Source: CAD feature listing. Evaluate the final solid. Frame: model axes, mm. A direction names the side the tool comes from. Coordinates: 2 decimals unless noted, no trailing zeros. Write each loop counter-clockwise with the first axis right and the second up, starting at its lowest first coordinate (ties: lowest second). Pieces come first, ordered by that corner, then holes. Notation, with made-up numbers: (25, -21) - (80, -21) arc R20 cw to (80, -3) - close; hole circle Ø2 at (42, 11). An arc over 180 degrees is marked (long way). One line per question, with ' | ' between items. Start each with the question number.
Q1. Cut plane D-D, the plane y = 1.1. Give the number of separate pieces and of enclosed holes in the cut face, plus the area to 3 significant figures.
Q2. Cut plane A-A, the plane z = 39. Return loops of the section in (x, y).
Q3. Line query: line 1 (X direction, y = 0.65, z = -74); line 2 (Z direction, x = 98, y = 1.5); line 3 (Z direction, x = -50.5, y = 2.4). Output: solid intervals per line, ascending.
Q4. Cut plane B-B, the plane z = -45. Return loops of the section in (x, y).
Q5. Access query for faces 1 (the face through (-26.74, 1.52, -95.9)), 2 (the face through (35.933, 1.521, -43.116)), 3 (the face through (22, 0, -5)). Directions: +Z, -Z, +X, -X, +Y, -Y. A direction counts if a zero-diameter tool reaches every point of the face in a straight line with its end or side. Return the directions, or none.
Q6. Cut plane C-C, the plane x = -64. Return loops of the section in (y, z), plus the area to 3 significant figures.
Q7. Draft query along Z for faces 4 (the face through (115.972, 1.521, 65.502)), 5 (the face through (68.61, 1.52, 89.45)), 6 (the face through (22, 3, -5)). Return one class per face: +Z half, -Z half, draft (parallel to the pull), parting line (faces both ways), or undercut.
Q8. Contact query for flat-ended pins moving along their axis: P1, Ø1.5, axis at x = 21, y = 1.5, coming from the -Z side; P2, Ø8.5, axis at x = -48.36, z = 94.35, coming from the -Y side; P3, Ø0.9, axis at x = 20.5, y = 1.5, coming from the +Z side. Output: stop coordinate, or through.
```python
from build123d import *

# Parameters (mm, degrees)
BOSS_EXTRUDE1_DEPTH = 3
BOSS_EXTRUDE2_DEPTH = 2
CUT_EXTRUDE4_DEPTH  = 167.076115532
SKETCH3_R           = 2.6
CUT_EXTRUDE5_DEPTH  = 167.076115532
CUT_EXTRUDE7_DEPTH  = 167.076115532
SKETCH11_R          = 1.6
CUT_EXTRUDE10_DEPTH = 10
SKETCH12_R          = 2.6
CUT_EXTRUDE12_DEPTH = 10
CUT_EXTRUDE13_DEPTH = 167.076115532


with BuildPart() as part:
    # Sketch1 → Boss-Extrude1 (new body)
    with BuildSketch(Plane(origin=(0, 0, 0), x_dir=(1, 0, 0), z_dir=(0, 1, 0))):
        Polygon((-59.316686906, 108.225499677), (101.185838411, 108.225499677), (125.934575753, 83.476762335), (125.934575753, -77.025762982), (101.185838411, -101.774500323), (-59.316686906, -101.774500323), (-84.065424247, -77.025762982), (-84.065424247, 83.476762335), align=None)
    extrude(amount=BOSS_EXTRUDE1_DEPTH)

    # Sketch2 → Boss-Extrude2 (add)
    with BuildSketch(Plane(origin=(0, 3, 0), x_dir=(1, 0, 0), z_dir=(0, 1, 0))):
        Polygon((-84.065424247, -77.025762982), (-45.174551282, -38.134890016), (-20.425813941, -62.883627358), (-59.316686906, -101.774500323), align=None)
        Polygon((125.934575753, -77.025762982), (93.880849872, -37.104770943), (66.751068905, -58.888061335), (101.185838411, -101.774500323), align=None)
        Polygon((101.185838411, 108.225499677), (62.16108336, 69.955487183), (86.665825958, 44.96747398), (125.934575753, 83.476762335), align=None)
        Polygon((-59.316686906, 108.225499677), (-24.100270952, 65.978558399), (-50.874640527, 43.659845911), (-84.065424247, 83.476762335), align=None)
    extrude(amount=-BOSS_EXTRUDE2_DEPTH)

    # Sketch7 → Cut-Extrude4 (cut, through all)
    with BuildSketch(Plane(origin=(0, 3, 0), x_dir=(1, 0, 0), z_dir=(0, 1, 0))):
        with BuildLine():
            ThreePointArc((-1.565424247, -17.674500323), (-2.696795097, -20.405871173), (0.034575753, -19.274500323))
            Line((0.034575753, -19.274500323), (-1.565424247, -19.274500323))
            Line((-1.565424247, -19.274500323), (-1.565424247, -17.674500323))
        make_face()
        with BuildLine():
            Line((-1.565424247, -19.274500323), (0.034575753, -19.274500323))
            ThreePointArc((0.034575753, -19.274500323), (-0.434053398, -18.143129473), (-1.565424247, -17.674500323))
            Line((-1.565424247, -17.674500323), (-1.565424247, -19.274500323))
        make_face()
        with BuildLine():
            ThreePointArc((43.434575753, -17.674500323), (42.303204903, -18.143129473), (41.834575753, -19.274500323))
            Line((41.834575753, -19.274500323), (43.434575753, -19.274500323))
            Line((43.434575753, -19.274500323), (43.434575753, -17.674500323))
        make_face()
        with BuildLine():
            Line((43.434575753, -19.274500323), (41.834575753, -19.274500323))
            ThreePointArc((41.834575753, -19.274500323), (43.434575753, -20.874500323), (45.034575753, -19.274500323))
            ThreePointArc((45.034575753, -19.274500323), (44.565946602, -18.143129473), (43.434575753, -17.674500323))
            Line((43.434575753, -17.674500323), (43.434575753, -19.274500323))
        make_face()
        with BuildLine():
            ThreePointArc((45.034575753, 25.725499677), (43.434575753, 27.325499677), (41.834575753, 25.725499677))
            Line((41.834575753, 25.725499677), (43.434575753, 25.725499677))
            Line((43.434575753, 25.725499677), (43.434575753, 24.125499677))
            ThreePointArc((43.434575753, 24.125499677), (44.565946602, 24.594128827), (45.034575753, 25.725499677))
        make_face()
        with BuildLine():
            Line((43.434575753, 25.725499677), (41.834575753, 25.725499677))
            ThreePointArc((41.834575753, 25.725499677), (42.303204903, 24.594128827), (43.434575753, 24.125499677))
            Line((43.434575753, 24.125499677), (43.434575753, 25.725499677))
        make_face()
        with BuildLine():
            ThreePointArc((-1.565424247, 24.125499677), (-0.434053398, 24.594128827), (0.034575753, 25.725499677))
            Line((0.034575753, 25.725499677), (-1.565424247, 25.725499677))
            Line((-1.565424247, 25.725499677), (-1.565424247, 24.125499677))
        make_face()
        with BuildLine():
            Line((-1.565424247, 25.725499677), (0.034575753, 25.725499677))
            ThreePointArc((0.034575753, 25.725499677), (-2.696795097, 26.856870527), (-1.565424247, 24.125499677))
            Line((-1.565424247, 24.125499677), (-1.565424247, 25.725499677))
        make_face()
    extrude(amount=-CUT_EXTRUDE4_DEPTH, mode=Mode.SUBTRACT)

    # Sketch3 → Cut-Extrude5 (cut, through all)
    with BuildSketch(Plane(origin=(0, 3, 0), x_dir=(1, 0, 0), z_dir=(0, 1, 0))):
        with Locations(Location((-27.143328362, 79.587675039, 0), (0, 0, 270))):
            Circle(SKETCH3_R)
        with Locations(Location((-55.427599609, 51.303403791, 0), (0, 0, 270))):
            Circle(SKETCH3_R)
        with Locations(Location((-76.640803045, 72.516607227, 0), (0, 0, 270))):
            Circle(SKETCH3_R)
        with Locations(Location((-48.356531798, 100.800878474, 0), (0, 0, 270))):
            Circle(SKETCH3_R)
        with Locations(Location((118.50995455, 72.516607227, 0), (0, 0, 90))):
            Circle(SKETCH3_R)
        with Locations(Location((97.296751114, 51.303403791, 0), (0, 0, 90))):
            Circle(SKETCH3_R)
        with Locations(Location((69.012479867, 79.587675039, 0), (0, 0, 90))):
            Circle(SKETCH3_R)
        with Locations(Location((90.225683303, 100.800878474, 0), (0, 0, 90))):
            Circle(SKETCH3_R)
        with Locations(Location((97.296751114, -44.852404438, 0), (0, 0, 270))):
            Circle(SKETCH3_R)
        with Locations(Location((118.50995455, -66.065607873, 0), (0, 0, 270))):
            Circle(SKETCH3_R)
        with Locations(Location((90.225683303, -94.349879121, 0), (0, 0, 270))):
            Circle(SKETCH3_R)
        with Locations(Location((69.012479867, -73.136675685, 0), (0, 0, 270))):
            Circle(SKETCH3_R)
        with Locations(Location((-27.143328362, -73.136675685, 0), (0, 0, 90))):
            Circle(SKETCH3_R)
        with Locations(Location((-55.427599609, -44.852404438, 0), (0, 0, 90))):
            Circle(SKETCH3_R)
        with Locations(Location((-76.640803045, -66.065607873, 0), (0, 0, 90))):
            Circle(SKETCH3_R)
        with Locations(Location((-48.356531798, -94.349879121, 0), (0, 0, 90))):
            Circle(SKETCH3_R)
    extrude(amount=-CUT_EXTRUDE5_DEPTH, mode=Mode.SUBTRACT)

    # Sketch9 → Cut-Extrude7 (cut, through all)
    with BuildSketch(Plane(origin=(0, 3, 0), x_dir=(1, 0, 0), z_dir=(0, 1, 0))):
        Polygon((-14.065424247, 83.225499677), (55.934575753, 83.225499677), (80.934575753, 108.225499677), (-39.065424247, 108.225499677), align=None)
        Polygon((-14.065424247, -76.774500323), (-39.065424247, -101.774500323), (80.934575753, -101.774500323), (55.934575753, -76.774500323), align=None)
    extrude(amount=-CUT_EXTRUDE7_DEPTH, mode=Mode.SUBTRACT)

    # Sketch11 → Cut-Extrude10 (cut)
    with BuildSketch(Plane(origin=(0, 3, 0), x_dir=(1, 0, 0), z_dir=(0, 1, 0))):
        with Locations(Location((-77.065424247, 17.565499677, 0), (0, 0, 270))):
            Circle(SKETCH11_R)
        with Locations(Location((-77.065424247, -11.114500323, 0), (0, 0, 270))):
            Circle(SKETCH11_R)
        with Locations(Location((-48.385424247, 17.565499677, 0), (0, 0, 270))):
            Circle(SKETCH11_R)
        with Locations(Location((-48.385424247, -11.114500323, 0), (0, 0, 90))):
            Circle(SKETCH11_R)
    extrude(amount=-CUT_EXTRUDE10_DEPTH, mode=Mode.SUBTRACT)

    # Sketch12 → Cut-Extrude12 (cut)
    with BuildSketch(Plane(origin=(0, 3, 0), x_dir=(1, 0, 0), z_dir=(0, 1, 0))):
        with Locations(Location((-34.065424247, 3.225499677, 0), (0, 0, 270))):
            Circle(SKETCH12_R)
        with Locations(Location((20.934575753, -51.774500323, 0), (0, 0, 270))):
            Circle(SKETCH12_R)
        with Locations(Location((75.934575753, 3.225499677, 0), (0, 0, 270))):
            Circle(SKETCH12_R)
        with Locations(Location((20.934575753, 58.225499677, 0), (0, 0, 270))):
            Circle(SKETCH12_R)
    extrude(amount=-CUT_EXTRUDE12_DEPTH, mode=Mode.SUBTRACT)

    # Sketch13 → Cut-Extrude13 (cut, through all)
    with BuildSketch(Plane(origin=(0, 3, 0), x_dir=(1, 0, 0), z_dir=(0, 1, 0))):
        with BuildLine():
            Line((10.934575753, -41.774500323), (30.934575753, -41.774500323))
            ThreePointArc((30.934575753, -41.774500323), (35.934575753, -36.774500323), (30.934575753, -31.774500323))
            Line((30.934575753, -31.774500323), (10.934575753, -31.774500323))
            ThreePointArc((10.934575753, -31.774500323), (5.934575753, -36.774500323), (10.934575753, -41.774500323))
        make_face()
        with BuildLine():
            Line((10.934575753, 38.225499677), (30.934575753, 38.225499677))
            ThreePointArc((30.934575753, 38.225499677), (35.934575753, 43.225499677), (30.934575753, 48.225499677))
            Line((30.934575753, 48.225499677), (10.934575753, 48.225499677))
            ThreePointArc((10.934575753, 48.225499677), (5.934575753, 43.225499677), (10.934575753, 38.225499677))
        make_face()
    extrude(amount=-CUT_EXTRUDE13_DEPTH, mode=Mode.SUBTRACT)


solid = part.part
```
Reply:
1) separate pieces: 1 | enclosed holes: 30 | area: 37,100 mm^2
2) outline: (-84.07, 0) - (6.46, 0) - (6.46, 3) - (-84.07, 3) - close; (35.41, 0) - (125.93, 0) - (125.93, 3) - (35.41, 3) - close
3) line 1: x = -84.07 to -78.78, -74.51 to 116.37, 120.65 to 125.93 | line 2: z = -108.23 to -53.81, -48.8 to 42.35, 47.36 to 101.77 | line 3: z = -108.23 to -102.27, -99.33 to 92.88, 95.82 to 101.77
4) outline: (-84.07, 0) - (6.26, 0) - (6.26, 3) - (-84.07, 3) - close; (35.61, 0) - (125.93, 0) - (125.93, 3) - (35.61, 3) - close
5) face 1: -Z, +Y, -Y | face 2: +Y, -Y | face 3: +Z, -Z, +X, -X, -Y
6) outline: (0, -103.54) - (3, -103.54) - (3, 97.09) - (0, 97.09) - close | area: 602 mm^2
7) face 4: undercut | face 5: +Z half | face 6: draft
8) P1: stops at z = -83.23 | P2: stops at y = 0 | P3: stops at z = 76.77
